Part print with two shaded views. Sizes in mm from the minimum x, y, z corner. A direction names the side the tool comes from. Give positions to 0.01 mm unless a question says otherwise; leave off trailing zeros. Write each loop counter-clockwise with the first axis right and the second up, starting at its lowest first coordinate (ties: lowest second). Pieces come first, ordered by that corner, then holes. Notation, with made-up numbers: (10.25, -22) -> (18.25, -22) arc R6 ccw to (18.25, -16) -> close; hole circle Ø4 at (-30.75, 15). An arc over 180 degrees is marked (long way). Answer in a Markdown table with one row per item. Add a question column.
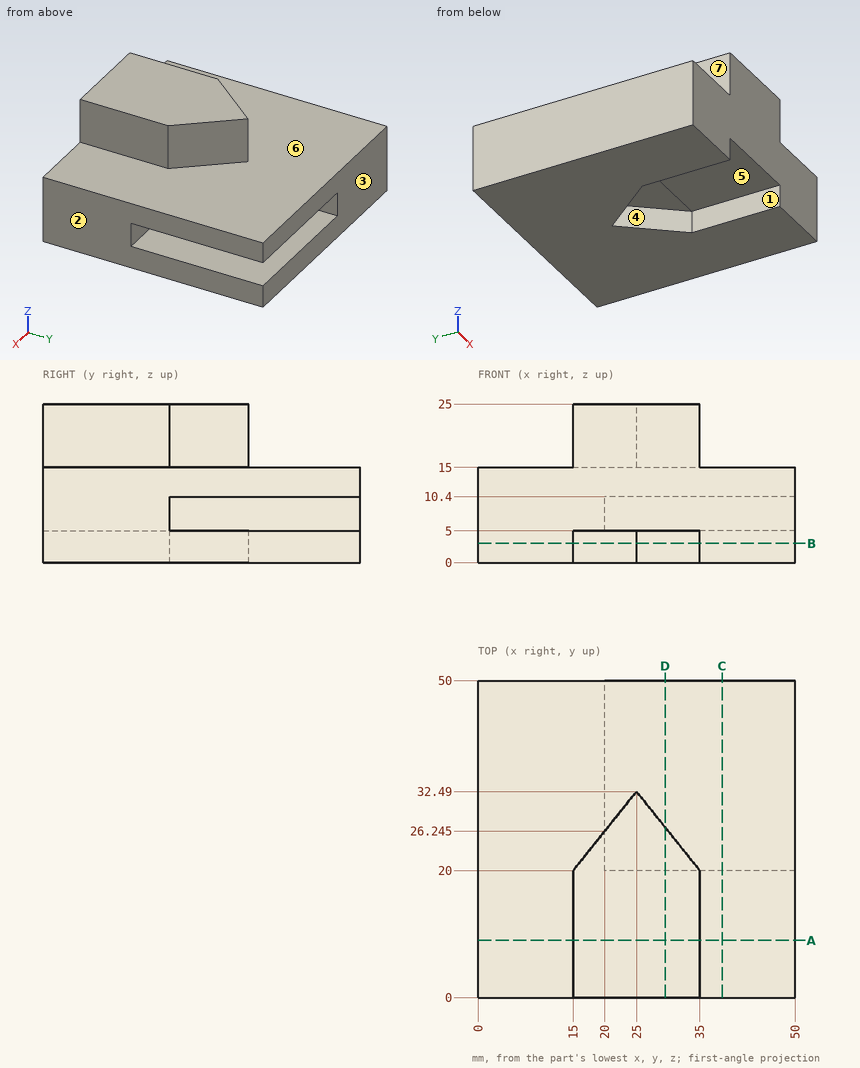
Item 1: Slice it at A-A, the plane y = 9. List the corners of the cut face in (x, z).
Item 2: Slice it at B-B, the plane z = 3. List the corners of the cut face in (x, y), then the cut area to 3 significant figures.
Item 3: Drop flat-ended pins along their axis: pin 1 Ø24 at (x, y) = (40, 35) entering from +Z; pin 2 Ø2.5 at (y, z) = (41.5, 8) entering from +X; pin 3 Ø8 at (y, z) = (10.5, 20.5) entering from +X. Give the stop position or say it passes through.
Item 4: Probe L1, parallel to Z at x = 45.5, y = 21.5; L2, parallel to Y at x = 34, z = 7.75; L3, parallel to Z at x = 31, y = 3. List the from-to ranges inside material, lowest first. Write a range as from..to.
Item 5: Mould opens along X. For the marked faces 1, 2, 3 and 4 say: released by +X, released by -X, zero draft, split by the parting line, or undercut.
Item 6: Which spindle directions (+Z, -Z, +X, -X, +Y, -Y) get a long thin tool onto all of the face, cutting with end or side? Do the marked faces 5, 6 and 7. Say none if no direction does.
Item 7: Slice it at D-D, the plane x = 29.5. List the corners of the cut face in (y, z), then the cut area to 3 significant figures.
Item 8: Slice it at C-C, the plane x = 38.5. List the corners of the cut face in (y, z).
Answer key:
| question | item | result |
|---|---|---|
| 1 | outline | (0, 0) -> (15, 0) -> (15, 5) -> (35, 5) -> (35, 0) -> (50, 0) -> (50, 15) -> (35, 15) -> (35, 25) -> (15, 25) -> (15, 15) -> (0, 15) -> close |
| 2 | outline | (0, 0) -> (15, 0) -> (15, 20) -> (25, 32.49) -> (35, 20) -> (35, 0) -> (50, 0) -> (50, 50) -> (0, 50) -> close |
| 2 | area | 1,980 mm² |
| 3 | pin 1 | stops at z = 15 |
| 3 | pin 2 | stops at x = 20 |
| 3 | pin 3 | stops at x = 35 |
| 4 | L1 | z = 0..5, 10.4..15 |
| 4 | L2 | y = 0..20 |
| 4 | L3 | z = 5..25 |
| 5 | face 1 | undercut |
| 5 | face 2 | released by +X |
| 5 | face 3 | zero draft |
| 5 | face 4 | undercut |
| 6 | face 5 | -Z, -Y |
| 6 | face 6 | +Z, +Y |
| 6 | face 7 | +Z, -X, +Y, -Y |
| 7 | outline | (0, 5) -> (20, 5) -> (20, 10.4) -> (50, 10.4) -> (50, 15) -> (26.87, 15) -> (26.87, 25) -> (0, 25) -> close; (26.87, 0) -> (50, 0) -> (50, 5) -> (26.87, 5) -> close |
| 7 | area | 722 mm² |
| 8 | outline | (0, 0) -> (50, 0) -> (50, 5) -> (20, 5) -> (20, 10.4) -> (50, 10.4) -> (50, 15) -> (0, 15) -> close |
